from build123d import *

# Parameters (mm, degrees)
SKETCH_1_W              = 36
SKETCH_1_H              = 9
BLOCKEXTRUDE_DEPTH      = 16
SKETCH_3_W              = 12.6
SKETCH_3_H              = 13
CLEVIS_SLOT_DEPTH       = 5
SKETCH_4_W              = 12.6
SKETCH_4_H              = 13
CUT_EXTRUDE_2_DEPTH     = 5
SKETCH_5_R              = 2.6
PIVOT_BORE_DEPTH        = 41.410394702
SKETCH_6_R              = 2.6
CUT_EXTRUDE_4_DEPTH     = 41.410394702
SKETCH_7_R              = 6.2
SPINDLE_CLEARANCE_DEPTH = 41.410394702


with BuildPart() as part:
    # 草图1 → BlockExtrude (new body)
    with BuildSketch(Plane.XY):
        with Locations((18, 4.5)):
            Rectangle(SKETCH_1_W, SKETCH_1_H)
    extrude(amount=BLOCKEXTRUDE_DEPTH)

    # 草图3 → Clevis_slot (cut, symmetric)
    with BuildSketch(Plane.XY.offset(8)):
        with Locations((4.3, 4.5)):
            Rectangle(SKETCH_3_W, SKETCH_3_H)
    extrude(amount=CLEVIS_SLOT_DEPTH, both=True, mode=Mode.SUBTRACT)

    # 草图4 → 切除-拉伸2 (cut, symmetric)
    with BuildSketch(Plane.XY.offset(8)):
        with Locations((31.7, 4.5)):
            Rectangle(SKETCH_4_W, SKETCH_4_H)
    extrude(amount=CUT_EXTRUDE_2_DEPTH, both=True, mode=Mode.SUBTRACT)

    # 草图5 → Pivot_bore (cut, through all)
    with BuildSketch(Plane.XY.offset(16)):
        with Locations((5, 4)):
            Circle(SKETCH_5_R)
    extrude(amount=-PIVOT_BORE_DEPTH, mode=Mode.SUBTRACT)

    # 草图6 → 切除-拉伸4 (cut, through all)
    with BuildSketch(Plane.XY.offset(16)):
        with Locations((31, 4)):
            Circle(SKETCH_6_R)
    extrude(amount=-CUT_EXTRUDE_4_DEPTH, mode=Mode.SUBTRACT)

    # 草图7 → Spindle_clearance (cut, through all)
    with BuildSketch(Plane(origin=(0, 9, 0), x_dir=(1, 0, 0), z_dir=(0, 1, 0))):
        with Locations(Location((18, -8, 0), (0, 0, 270))):
            Circle(SKETCH_7_R)
    extrude(amount=-SPINDLE_CLEARANCE_DEPTH, mode=Mode.SUBTRACT)


solid = part.part
Geometry check sheet. Reference: the model listing, model coordinates, mm. A direction names the side the tool comes from. Round coordinates to 2 decimals unless told otherwise and drop trailing zeros. Order: outer loops, then holes, each group sorted by start corner. A loop starts at its lowest first (then second) coordinate and runs counter-clockwise, first axis right, second up. Notation, with made-up numbers: M 3.5,-7.75 L 9.5,-7.75 A19 ccw 9.5,19.25 Z; hole C 50.5,-40 d2. An arc over 180 degrees is marked long. Answer in a Markdown table with one row per item. Add a question column.
Item 1: Depth check by flat-ended pin: pin 1 Ø2.5 at (y, z) = (6, 6.5) entering from -X. Enter the tip coordinate at first touch or a pass-through.
Item 2: Sectioned sample at A-A, the plane x = 18. Enter the section's corners in (y, z).
Item 3: Set-up check for faces 1 (the face through (28.4, 4.1, 1.5)), 2 (the face through (29, 7, 13)), 3 (the face through (6, 7, 3)): record each of +Z, -Z, +X, -X, +Y, -Y from which the full face is reachable in a straight line by a thin tool's end or side.
Item 4: Sectioned sample at D-D, the plane y = 3.5. State how many separate pieces and enclosed holes the cut face has, plus the area to 3 significant figures.
Item 5: Material ranges on L1, parallel to Z at x = 26.5, y = 4.75; L2, parallel to Y at x = 31, z = 13.6; L3, parallel to X at y = 6.5, z = 8, recorded low to high. Write a range as [from, to].
Item 6: Sectioned sample at B-B, the plane x = 5. Enter the section's corners in (y, z).
Item 7: Sectioned sample at C-C, the plane z = 8. Enter the section's corners in (x, y).
Item 8: Draft check along Y on faces 4 (the face through (36, 4, 1)), 5 (the face through (22, 0, 13)), 6 (the face through (4.662, 6.578, 14.521)). Enter one of: released by +Y, released by -Y, zero draft, split by the parting line, or undercut.
Filled in:
| question | item | result |
|---|---|---|
| 1 | pin 1 | stops at x = 10.6 |
| 2 | outline | M 0,0 L 9,0 L 9,1.8 L 0,1.8 Z; M 0,14.2 L 9,14.2 L 9,16 L 0,16 Z |
| 3 | face 1 | +Z, -Z |
| 3 | face 2 | +X, +Y, -Y |
| 3 | face 3 | -X, +Y, -Y |
| 4 | separate pieces | 5 |
| 4 | enclosed holes | 1 |
| 4 | area | 182 mm² |
| 5 | L1 | z = [0, 3], [13, 16] |
| 5 | L2 | y = [0, 1.4], [6.6, 9] |
| 5 | L3 | x = [10.6, 11.8], [24.2, 25.4] |
| 6 | outline | M 0,0 L 1.4,0 L 1.4,3 L 0,3 Z; M 0,13 L 1.4,13 L 1.4,16 L 0,16 Z; M 6.6,0 L 9,0 L 9,3 L 6.6,3 Z; M 6.6,13 L 9,13 L 9,16 L 6.6,16 Z |
| 7 | outline | M 10.6,0 L 11.8,0 L 11.8,9 L 10.6,9 Z; M 24.2,0 L 25.4,0 L 25.4,9 L 24.2,9 Z |
| 8 | face 4 | zero draft |
| 8 | face 5 | released by -Y |
| 8 | face 6 | undercut |
